For this review, take the finished solid that the model builds, in its own axes (mm). Face numbers are marked on the shaded views. A direction names the side the tool comes from. Coordinates: 2 decimals unless noted, no trailing zeros. Loops run counter-clockwise (first coordinate to the right, second up) from the corner with the lowest first, then second, coordinate; pieces in that order, holes last. Notation, with made-up numbers: M 11.5,-18 L 44.5,-18 A11 cw 44.5,-5 Z; hole C -23.75,73 d9. An arc over 180 degrees is marked long. Write item = value, one per line.
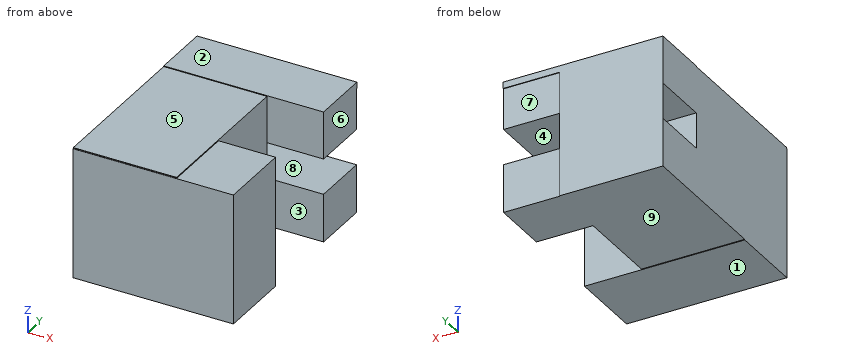
from build123d import *

# Parameters (mm, degrees)
F0_W     = 118.5401678085
F0_H     = 70.9766112268
F1_DEPTH = 56.134
F2_W     = 40.3737127781
F2_H     = 70.7922605798
F3_DEPTH = 87.122
F4_W     = 31.5654948354
F4_H     = 3.5027423874
F4_W_2   = 0.3687143326
F4_H_2   = 67.8425794467
F5_DEPTH = 86.868
F6_W     = 31.7498482764
F6_H     = 19.3572575226
F7_DEPTH = 92.71


with BuildPart() as f1:
    # F0 (on Right) → F1 (new body)
    with BuildSketch(Plane.YZ):
        with Locations((-27.3358747363, -19.541611895)):
            Rectangle(F0_W, F0_H)
    extrude(amount=F1_DEPTH)

    # F2 (on Right) → F3 (join)
    with BuildSketch(Plane.YZ):
        with Locations((-66.6034594178, -20.0025015511)):
            Rectangle(F2_W, F2_H)
    extrude(amount=F3_DEPTH)

    # F4 (on Right) → F5 (join)
    with BuildSketch(Plane.YZ):
        with Locations((15.7827474177, 14.564033132)):
            Rectangle(F4_W, F4_H)
        with Locations((31.7498520017, 14.564033132)):
            Rectangle(F4_W_2, F4_H)
        with Locations((15.7827474177, -21.108627785)):
            Rectangle(F4_W, F4_H_2)
    extrude(amount=F5_DEPTH)

    # F6 (on Right) → F7 (cut)
    with BuildSketch(Plane.YZ):
        with Locations((15.8749241382, -19.1729026847)):
            Rectangle(F6_W, F6_H)
    extrude(amount=F7_DEPTH, mode=Mode.SUBTRACT)


solid = f1.part
Q1. For line 1 along Y through (x, z) = (63.5, -48.5); line 2 along Z through (x, y) = (58, 10.5); line 3 along Z through (x, y) = (64, -50), list the stretches that pass through material, from the lowest coordinate up.
Solved:
line_1 = -86.79 to -46.42, 0 to 31.57
line_2 = -55.03 to -28.85, -9.49 to 16.32
line_3 = -55.4 to 15.39
Q2. Add section D-D (z = 10.5). Write out the cut boundary in (x, y).
Solved:
outline = M 0,-86.79 L 87.12,-86.79 L 87.12,-46.42 L 56.13,-46.42 L 56.13,0 L 86.87,0 L 86.87,31.57 L 56.13,31.57 L 56.13,31.93 L 0,31.93 Z
Q3. Machinability: for the marked faces 5, 6, 7, 8 and 9, which of the approach directions +Z, -Z, +X, -X, +Y, -Y give a long, thin tool a straight path to every point of the face, cutting with its end or side? Answer none if there is none.
Solved:
face_5 = +Z, +X, -X, -Y
face_6 = +Z, -Z, +X, +Y
face_7 = -Z, +X, +Y
face_8 = +X, -X
face_9 = -Z, +X, -X, +Y
Q4. Draft analysis for pull direction Z (two halves, no side actions). For the marked faces 1, 2, 3 and 4, state which applies: +Z half, -Z half, draft (parallel to the pull), parting line (faces both ways), or undercut.
Solved:
face_1 = -Z half
face_2 = +Z half
face_3 = draft
face_4 = undercut
Q5. Add section C-C (y = 21.5). Write out the cut boundary in (x, z), and give its area (3 significant figures).
Solved:
outline = M 0,-55.03 L 86.87,-55.03 L 86.87,-28.85 L 0,-28.85 Z; M 0,-9.49 L 86.87,-9.49 L 86.87,16.32 L 0,16.32 Z
area = 4,520 mm²
Q6. Add section B-B (x = 69). Write out the cut boundary in (y, z), and give its area (3 significant figures).
Solved:
outline = M -86.79,-55.4 L -46.42,-55.4 L -46.42,15.39 L -86.79,15.39 Z; M 0,-55.03 L 31.57,-55.03 L 31.57,-28.85 L 0,-28.85 Z; M 0,-9.49 L 31.57,-9.49 L 31.57,12.81 L 31.93,12.81 L 31.93,16.32 L 0,16.32 Z
area = 4,500 mm²
Q7. For pin 1 Ø9.5 at (x, y) = (40, 17.5) entering from -Z; pin 2 Ø13 at (y, z) = (13, -42) entering from +X; pin 3 Ø10 at (x, y) = (39.5, -43.5) entering from +Z; pin 4 Ø24.5 at (x, z) = (72, 1) entering from +Y, all flat-tipped, find the tip position at first contact; note any pin that passes through.
Solved:
pin_1 = -55.03
pin_2 = 86.87
pin_3 = 15.95
pin_4 = 31.93
Q8. Add section A-A (z = -15). Write out the cut boundary in (x, y), and give its area (3 significant figures).
Solved:
outline = M 0,-86.79 L 87.12,-86.79 L 87.12,-46.42 L 56.13,-46.42 L 56.13,0 L 0,0 Z; M 0,31.75 L 56.13,31.75 L 56.13,31.93 L 0,31.93 Z
area = 6,130 mm²
